Model file for the job. Use its own axes, mm. Coordinates: 2 decimals unless noted, no trailing zeros. Order: outer loops, then holes, each group sorted by start corner. A loop starts at its lowest first (then second) coordinate and runs counter-clockwise, first axis right, second up. Notation, with made-up numbers: (8.25, -39.5) -> (21.25, -39.5) arc R18 cw to (21.25, -35.5) -> close; hole circle Ø7 at (9, -11.75). An arc over 180 degrees is marked (long way). Use CSV: the item, a comma, the result in double quotes. Start each with the question number.
(1) Cut at B-B on x = 464.5. Write the cut outline in (y, z).
(2) Probe L1, parallel to Y at x = 200, z = 8.5; L2, parallel to X at y = 11, z = 11.75; L3, parallel to X at y = 74, z = 6.25. List the from-to ranges inside material, lowest first.
(3) Cut at A-A on z = 7. Write the cut outline in (x, y).
(4) Cut at C-C on x = 69. Write the cut outline in (y, z).
(5) Pin check, flat tips, straight feed: pin 1 Ø3 at (x, z) = (198.5, 7.5) entering from -Y; pin 2 Ø1.5 at (x, z) = (153, 3.5) entering from +Y; pin 3 Ø8 at (x, z) = (104, 10) entering from +Y. Stop position of each tip, or through.
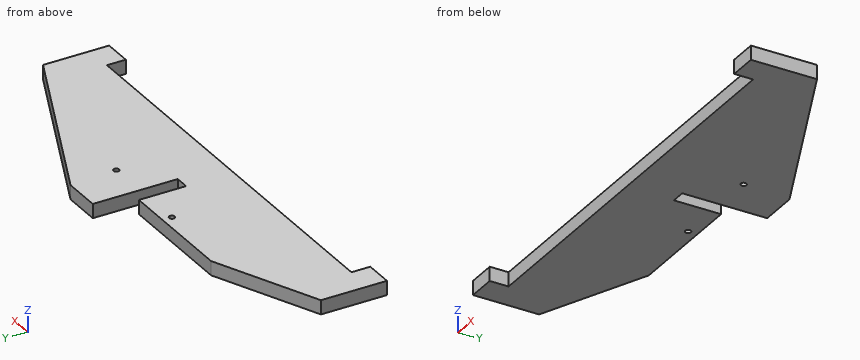
```python
from build123d import *

# Parameters (mm, degrees)
ESQUISSE1_R        = 3
BOSS_EXTRU_1_DEPTH = 15


with BuildPart() as part:
    # Esquisse1 → Boss.-Extru.1 (new body)
    with BuildSketch(Plane.XY):
        Polygon((0, 0), (30, 0), (30, 20), (470, 20), (470, 0), (500, 0), (500, 70), (297.5, 160), (257.5, 160), (257.5, 70), (242.5, 70), (242.5, 120), (112.5, 120), (0, 70), align=None)
        with Locations((200, 110)):
            Circle(ESQUISSE1_R, mode=Mode.SUBTRACT)
        with Locations((300, 110)):
            Circle(ESQUISSE1_R, mode=Mode.SUBTRACT)
    extrude(amount=BOSS_EXTRU_1_DEPTH)


solid = part.part
```
Outcome:
1,outline,"(20, 0) -> (85.78, 0) -> (85.78, 15) -> (20, 15) -> close"
2,L1,"20 to 107, 113 to 120"
2,L2,"0 to 30, 470 to 500"
2,L3,"9 to 242.5, 257.5 to 491"
3,outline,"(0, 0) -> (30, 0) -> (30, 20) -> (470, 20) -> (470, 0) -> (500, 0) -> (500, 70) -> (297.5, 160) -> (257.5, 160) -> (257.5, 70) -> (242.5, 70) -> (242.5, 120) -> (112.5, 120) -> (0, 70) -> close; hole circle Ø6 at (200, 110); hole circle Ø6 at (300, 110)"
4,outline,"(20, 0) -> (100.67, 0) -> (100.67, 15) -> (20, 15) -> close"
5,pin 1,"y = 20"
5,pin 2,"y = 120"
5,pin 3,"y = 118"
